For this review, take the finished solid that the model builds, in its own axes (mm). Give positions to 0.01 mm unless a question says otherwise; leave off trailing zeros. Loops run counter-clockwise (first coordinate to the right, second up) from the corner with the lowest first, then second, coordinate; pieces in that order, holes last. Notation, with made-up numbers: M 5.25,-26.75 L 31.25,-26.75 A29 cw 31.25,7.25 Z; hole C 23.25,45 d11. An arc over 180 degrees is marked long. Use CSV: the item, a comma, the result in double quotes. Start each with the question number.
1. Take a section at C-C, the plane y = 1.2. State how many separate pieces and enclosed holes the cut face has, and give its area (3 significant figures).
2. Take a section at B-B, the plane z = 11.5. Write out the cut boundary in (x, y), and give its area (3 significant figures).
3. Take a section at A-A, the plane x = 11.5. Write out the cut boundary in (y, z), and give its area (3 significant figures).
4. To check wall thickness, follow line 1 (X direction, y = 0.8, z = 11.5); line 2 (X direction, y = 0.7, z = -11); line 3 (X direction, y = 0.5, z = 10). State the ranges of each line that lie inside material, in increasing order. Write a range as [from, to].
5. Take a section at D-D, the plane z = -20. Write out the cut boundary in (x, y).
6. Insertion check: P1, Ø0.5, axis at x = 21.5, y = 1, coming from the -Z side; P2, Ø0.5, axis at x = -22.5, y = 1, coming from the +Z side; P3, Ø0.9, axis at x = 9.48, z = -9.48, coming from the +Y side. Each pin has a flat end and moves straight along its axis. Give the tip position at first contact, or say it passes through.
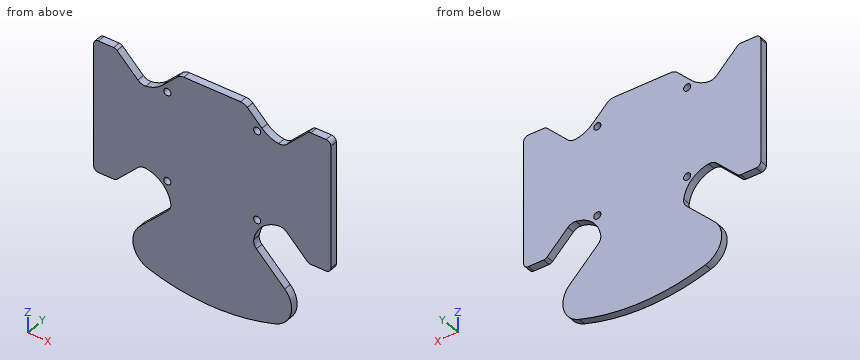
from build123d import *

# Parameters (mm, degrees)
SKETCH1_R           = 0.75
BOSS_EXTRUDE1_DEPTH = 1.6


with BuildPart() as part:
    # Sketch1 → Boss-Extrude1 (new body)
    with BuildSketch(Plane(origin=(0, 0, 0), x_dir=(1, 0, 0), z_dir=(0, 1, 0))):
        with BuildLine():
            Line((-20.071067812, -13.707106781), (-15.681770053, -9.317809022))
            ThreePointArc((-15.681770053, -9.317809022), (-14.907327841, -8.837110286), (-14, -8.75))
            ThreePointArc((-14, -8.75), (-12.101565565, -9.330988792), (-10.488732177, -10.488732177))
            Line((-10.488732177, -10.488732177), (-7.402704805, -13.57475955))
            ThreePointArc((-7.402704805, -13.57475955), (-6.753858107, -14.008305053), (-5.988491243, -14.160545988))
            Line((-5.988491243, -14.160545988), (5.988491243, -14.160545988))
            ThreePointArc((5.988491243, -14.160545988), (6.753858107, -14.008305053), (7.402704805, -13.57475955))
            Line((7.402704805, -13.57475955), (10.488732177, -10.488732177))
            ThreePointArc((10.488732177, -10.488732177), (12.101565565, -9.330988792), (14, -8.75))
            ThreePointArc((14, -8.75), (14.907327841, -8.837110286), (15.681770053, -9.317809022))
            Line((15.681770053, -9.317809022), (20.071067812, -13.707106781))
            ThreePointArc((20.071067812, -13.707106781), (20.395491161, -13.923879533), (20.778174593, -14))
            Line((20.778174593, -14), (24, -14))
            ThreePointArc((24, -14), (24.707106781, -13.707106781), (25, -13))
            Line((25, -13), (25, 13))
            ThreePointArc((25, 13), (24.707106781, 13.707106781), (24, 14))
            Line((24, 14), (20.778174593, 14))
            ThreePointArc((20.778174593, 14), (20.395491161, 13.923879533), (20.071067812, 13.707106781))
            Line((20.071067812, 13.707106781), (15.681770053, 9.317809022))
            ThreePointArc((15.681770053, 9.317809022), (14.907327841, 8.837110286), (14, 8.75))
            ThreePointArc((14, 8.75), (10.488732177, 10.488732177), (8.75, 14))
            ThreePointArc((8.75, 14), (8.837110286, 14.907327841), (9.317809022, 15.681770053))
            Line((9.317809022, 15.681770053), (15.27484739, 21.638808421))
            ThreePointArc((15.27484739, 21.638808421), (16.603119619, 26.333389297), (13.300387568, 29.924399979))
            ThreePointArc((13.300387568, 29.924399979), (0, 32.053914601), (-13.300387568, 29.924399979))
            ThreePointArc((-13.300387568, 29.924399979), (-16.603119619, 26.333389297), (-15.27484739, 21.638808421))
            Line((-15.27484739, 21.638808421), (-9.317809022, 15.681770053))
            ThreePointArc((-9.317809022, 15.681770053), (-8.837110286, 14.907327841), (-8.75, 14))
            ThreePointArc((-8.75, 14), (-10.488732177, 10.488732177), (-14, 8.75))
            ThreePointArc((-14, 8.75), (-14.907327841, 8.837110286), (-15.681770053, 9.317809022))
            Line((-15.681770053, 9.317809022), (-20.071067812, 13.707106781))
            ThreePointArc((-20.071067812, 13.707106781), (-20.395491161, 13.923879533), (-20.778174593, 14))
            Line((-20.778174593, 14), (-24, 14))
            ThreePointArc((-24, 14), (-24.707106781, 13.707106781), (-25, 13))
            Line((-25, 13), (-25, -13))
            ThreePointArc((-25, -13), (-24.707106781, -13.707106781), (-24, -14))
            Line((-24, -14), (-20.778174593, -14))
            ThreePointArc((-20.778174593, -14), (-20.395491161, -13.923879533), (-20.071067812, -13.707106781))
        make_face()
        with Locations(Location((-9.475230868, 9.475230868, 0), (0, 0, 270))):
            Circle(SKETCH1_R, mode=Mode.SUBTRACT)
        with Locations(Location((9.475230868, -9.475230868, 0), (0, 0, 270))):
            Circle(SKETCH1_R, mode=Mode.SUBTRACT)
        with Locations(Location((9.475230868, 9.475230868, 0), (0, 0, 270))):
            Circle(SKETCH1_R, mode=Mode.SUBTRACT)
        with Locations(Location((-9.475230868, -9.475230868, 0), (0, 0, 270))):
            Circle(SKETCH1_R, mode=Mode.SUBTRACT)
    extrude(amount=BOSS_EXTRUDE1_DEPTH)


solid = part.part
Result set:
1,separate pieces,"1"
1,enclosed holes,"4"
1,area,"1,710 mm2"
2,outline,"M -25,0 L -17.86,0 L -17.86,1.6 L -25,1.6 Z; M -9.48,0 L 9.48,0 L 9.48,1.6 L -9.48,1.6 Z; M 17.86,0 L 25,0 L 25,1.6 L 17.86,1.6 Z"
2,area,"53.2 mm2"
3,outline,"M 0,-30.47 L 1.6,-30.47 L 1.6,-17.86 L 0,-17.86 Z; M 0,-9.67 L 1.6,-9.67 L 1.6,9.67 L 0,9.67 Z"
3,area,"51.1 mm2"
4,line 1,"[-25, -17.86], [-9.48, 9.48], [17.86, 25]"
4,line 2,"[-25, -17.36], [-10.03, 10.03], [17.36, 25]"
4,line 3,"[-25, -16.36], [-11.04, -10.01], [-8.94, 8.94], [10.01, 11.04], [16.36, 25]"
5,outline,"M -13.64,0 L 13.64,0 L 13.64,1.6 L -13.64,1.6 Z"
6,P1,"z = -14"
6,P2,"z = 14"
6,P3,"through"
